Input: dimensioned drawing with shaded views. Units: mm. Origin: part minimum x, y, z. A direction names the side the tool comes from. Coordinates: 2 decimals unless noted, no trailing zeros. Loops run counter-clockwise (first coordinate to the right, second up) from the corner with the lowest first, then second, coordinate; pieces in that order, holes last.
Item 1: Pin query (flat end, axial travel): pin 1 Ø5 at (x, z) = (19, 66.5) entering from -Y; pin 2 Ø8 at (y, z) = (27, 23.5) entering from -X; pin 3 Ø4 at (y, z) = (13, 86.5) entering from +X; pin 4 Ø4 at (y, z) = (27.5, 29.5) entering from +X. Return the tip coordinate at first contact, or that it passes through.
Item 2: Section query A-A, the plane x = 74.5. Return the cut outline in (y, z) (3 decimals), then the cut area to 3 significant figures.
Item 3: Reachability of the marked faces 5 and 6 from +Z, -Z, +X, -X, +Y, -Y: full face, straight path, thin tool, end or side. Return the list, or none.
Item 4: Section query D-D, the plane z = 33.5. Return the cut outline in (x, y) (1 decimal), then the cut area to 3 significant figures.
Item 5: Line query: probe 1 along Y at (x, z) = (61, 74); probe 2 along X at (y, z) = (20.5, 23); probe 3 along Z at (x, y) = (82, 32). Output: solid intervals per line, ascending.
Item 6: Section query B-B, the plane z = 69. Return the cut outline in (x, y).
Item 7: Section query C-C, the plane y = 34. Return the cut outline in (x, z).
Item 8: Pull-direction query (Y, two-part tool) for the marked faces 1, 2, 3 and 4; classes: +Y half, -Y half, draft (parallel to the pull), parting line (faces both ways), or undercut.
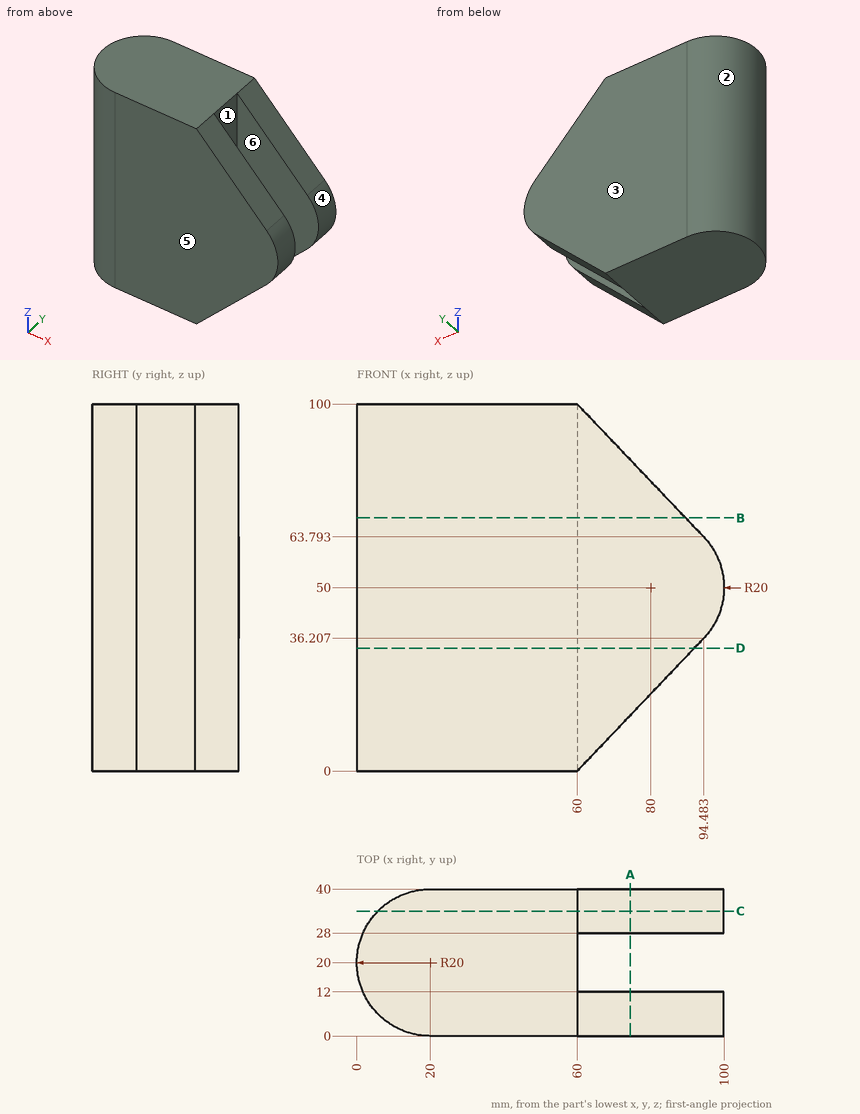
Verdict:
1. pin 1: stops at y = 0
1. pin 2: stops at x = 0.23
1. pin 3: stops at x = 74.51
1. pin 4: stops at x = 89.94
2. outline: (0, 15.225) - (12, 15.225) - (12, 84.775) - (0, 84.775) - close; (28, 15.225) - (40, 15.225) - (40, 84.775) - (28, 84.775) - close
2. area: 1,670 mm2
3. face 5: +Z, -Z, +X, -X, -Y
3. face 6: +Z, -Z, +X
4. outline: (20, 0) - (91.9, 0) - (91.9, 12) - (60, 12) - (60, 28) - (91.9, 28) - (91.9, 40) - (20, 40) arc R20 ccw to start
4. area: 2,990 mm2
5. probe 1: y = 0 to 12, 28 to 40
5. probe 2: x = 0.01 to 60
5. probe 3: z = 23.1 to 76.9
6. outline: (20, 0) - (89.52, 0) - (89.52, 12) - (60, 12) - (60, 28) - (89.52, 28) - (89.52, 40) - (20, 40) arc R20 ccw to start
7. outline: (5.72, 0) - (60, 0) - (94.48, 36.21) arc R20 ccw to (94.48, 63.79) - (60, 100) - (5.72, 100) - close
8. face 1: undercut
8. face 2: parting line
8. face 3: +Y half
8. face 4: draft
